Check sheet for the modelled part. Datum: model origin and axes. Units: mm. Face numbers are marked on the shaded views. A direction names the side the tool comes from. Coordinates: 2 decimals unless noted, no trailing zeros. Write each loop counter-clockwise with the first axis right and the second up, starting at its lowest first coordinate (ties: lowest second). Pieces come first, ordered by that corner, then holes. Notation, with made-up numbers: (82.25, -33.5) -> (102.25, -33.5) arc R13 ccw to (102.25, -17.5) -> close; hole circle Ø11 at (-37, -30.5). An arc over 180 degrees is marked (long way). One line per item, written item: value. Start each with the question number.
1) Set-up check for the marked faces 1, 2 and 3: record each of +Z, -Z, +X, -X, +Y, -Y from which the full face is reachable in a straight line by a thin tool's end or side.
2) Draft check along X on the marked faces 4, 5, 6 and 7. Enter one of: +X half, -X half, draft (parallel to the pull), parting line (faces both ways), or undercut.
3) Gauge pin test, flat ends, axial feed: P1, Ø8, axis at y = -39.5, z = 43.5, coming from the -X side; P2, Ø1, axis at y = -33, z = 13, coming from the +X side; P3, Ø12, axis at y = 5, z = 49.5, coming from the +X side; P4, Ø1, axis at x = -4.5, z = 30.5, coming from the -Y side. Record the tip position at first contact, or that the pin passes through.
4) Sectioned sample at A-A on z = 25. Enter the section's corners in (x, y), plus the area to 3 significant figures.
5) Sectioned sample at B-B on x = 32. Enter the section's corners in (y, z), plus the area to 3 significant figures.
6) Sectioned sample at D-D on x = -22. Enter the section's corners in (y, z), plus the area to 3 significant figures.
7) Sectioned sample at C-C on y = -16. Enter the section's corners in (x, z), plus the area to 3 significant figures.
8) Scan lines: line 1 along Y through (x, z) = (-32, 10); line 2 along X through (y, z) = (-11, 25); line 3 along X through (y, z) = (48, 12). Record each from-to range of solid material in increasing order. Write a range as [from, to].
```python
from build123d import *

# Parameters (mm, degrees)
ESQUISSE1_W                  = 80
ESQUISSE1_H                  = 112
BOSS_EXTRU_1_DEPTH           = 100
ESQUISSE4_R                  = 2.5
ENL_V_MAT_EXTRU_2_DEPTH      = 100
ENL_V_MAT_EXTRU_2_DEPTH_BACK = 1
BOSS_EXTRU_2_DEPTH           = 112
BOSS_EXTRU_4_DEPTH           = 112
ENL_V_MAT_EXTRU_6_DEPTH      = 112
ESQUISSE16_R                 = 4.25
ENL_V_MAT_EXTRU_7_DEPTH      = 112
ESQUISSE15_R                 = 4.25
ENL_V_MAT_EXTRU_10_DEPTH     = 112
CONG_1_R                     = 10
CONG_2_R                     = 5
ESQUISSE17_R                 = 4.5
ENL_V_MAT_EXTRU_12_DEPTH     = 112


with BuildPart() as part:
    # Esquisse1 → Boss.-Extru.1 (new body)
    with BuildSketch(Plane.XY):
        Rectangle(ESQUISSE1_W, ESQUISSE1_H)
    extrude(amount=BOSS_EXTRU_1_DEPTH)

    # Esquisse4 → Enlèv. mat.-Extru.2 (cut, two sides)
    with BuildSketch(Plane.XY) as enl_v_mat_extru_2_sk:
        with Locations((-32, 47.99765818)):
            Circle(ESQUISSE4_R)
        with Locations((32, 48)):
            Circle(ESQUISSE4_R)
        with Locations((-32, -48)):
            Circle(ESQUISSE4_R)
        with Locations((32, -48)):
            Circle(ESQUISSE4_R)
    extrude(amount=ENL_V_MAT_EXTRU_2_DEPTH, mode=Mode.SUBTRACT)
    extrude(enl_v_mat_extru_2_sk.sketch, amount=-ENL_V_MAT_EXTRU_2_DEPTH_BACK, mode=Mode.SUBTRACT)

    # Esquisse11 → Boss.-Extru.2 (add)
    with BuildSketch(Plane(origin=(0, 56, 0), x_dir=(1, 0, 0), z_dir=(0, 1, 0))):
        Polygon((-60, -65), (0, -5), (60, -65), align=None)
    extrude(amount=-BOSS_EXTRU_2_DEPTH)

    # Esquisse13 → Boss.-Extru.4 (add)
    with BuildSketch(Plane(origin=(0, 56, 0), x_dir=(1, 0, 0), z_dir=(0, 1, 0))):
        Polygon((-60, -65), (-40, -85), (-40, -65), align=None)
        Polygon((60, -65), (40, -85), (40, -65), align=None)
    extrude(amount=-BOSS_EXTRU_4_DEPTH)

    # Esquisse14 → Enlèv. mat.-Extru.6 (cut)
    with BuildSketch(Plane(origin=(0, 56, 0), x_dir=(1, 0, 0), z_dir=(0, 1, 0))):
        Polygon((-50, -75), (0, -25), (50, -75), (40, -85), (40, -100), (-40, -100), (-40, -85), align=None)
    extrude(amount=-ENL_V_MAT_EXTRU_6_DEPTH, mode=Mode.SUBTRACT)

    # Esquisse16 → Enlèv. mat.-Extru.7 (cut)
    with BuildSketch(Plane(origin=(2.5, 0, 2.5), x_dir=(-0.707106781, 0, 0.707106781), z_dir=(-0.707106781, 0, -0.707106781))):
        with Locations((74.388347648, 36)):
            Circle(ESQUISSE16_R)
        with Locations((74.388347648, -36)):
            Circle(ESQUISSE16_R)
    extrude(amount=-ENL_V_MAT_EXTRU_7_DEPTH, mode=Mode.SUBTRACT)

    # Esquisse15 → Enlèv. mat.-Extru.10 (cut)
    with BuildSketch(Plane(origin=(-2.5, 0, 2.5), x_dir=(-0.707106781, 0, -0.707106781), z_dir=(0.707106781, 0, -0.707106781))):
        with Locations((-74.388347648, 36)):
            Circle(ESQUISSE15_R)
        with Locations((-74.388347648, -36)):
            Circle(ESQUISSE15_R)
    extrude(amount=-ENL_V_MAT_EXTRU_10_DEPTH, mode=Mode.SUBTRACT)

    # Congé1
    cong_1_edges = [part.edges().sort_by_distance(p)[0] for p in [
        (-55, -56, 70),
        (-55, 56, 70),
        (55, 56, 70),
        (55, -56, 70),
    ]]
    fillet(cong_1_edges, radius=CONG_1_R)

    # Congé2
    cong_2_edges = [part.edges().sort_by_distance(p)[0] for p in [
        (40, -56, 22.5),
        (-40, -56, 22.5),
        (-40, 56, 22.5),
        (40, 56, 22.5),
    ]]
    fillet(cong_2_edges, radius=CONG_2_R)

    # Esquisse17 → Enlèv. mat.-Extru.12 (cut)
    with BuildSketch(Plane(origin=(0, 56, 0), x_dir=(1, 0, 0), z_dir=(0, 1, 0))):
        with Locations((0, -25)):
            Circle(ESQUISSE17_R)
    extrude(amount=-ENL_V_MAT_EXTRU_12_DEPTH, mode=Mode.SUBTRACT)


solid = part.part
```
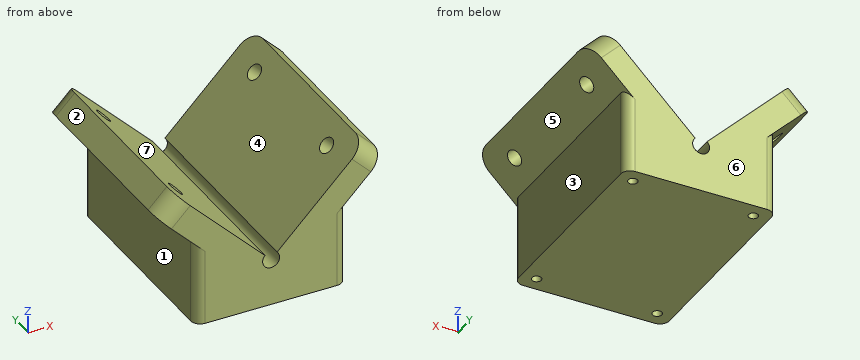
Answers:
1. face 1: -Z, -X, +Y, -Y
1. face 2: +Z, -X, +Y, -Y
1. face 3: -Z, +X, +Y, -Y
2. face 4: undercut
2. face 5: +X half
2. face 6: draft
2. face 7: undercut
3. P1: stops at x = -42.5
3. P2: stops at x = 40
3. P3: stops at x = 50.5
3. P4: passes through
4. outline: (-40, -51) arc R5 ccw to (-35, -56) -> (-4.5, -56) -> (-4.5, 56) -> (-35, 56) arc R5 ccw to (-40, 51) -> close; (4.5, -56) -> (35, -56) arc R5 ccw to (40, -51) -> (40, 51) arc R5 ccw to (35, 56) -> (4.5, 56) -> close; hole circle Ø5 at (-32, -48); hole circle Ø5 at (-32, 48); hole circle Ø5 at (32, -48); hole circle Ø5 at (32, 48)
4. area: 7,850 mm2
5. outline: (-56, 0) -> (-50.5, 0) -> (-50.5, 37) -> (-45.5, 37) -> (-45.5, 0) -> (45.5, 0) -> (45.5, 37) -> (50.5, 37) -> (50.5, 0) -> (56, 0) -> (56, 57) -> (-56, 57) -> close
5. area: 6,010 mm2
6. outline: (-56, 0) -> (56, 0) -> (56, 47) -> (-56, 47) -> close
6. area: 5,260 mm2
7. outline: (-60, 65) -> (-40, 45) -> (-40, 0) -> (40, 0) -> (40, 45) -> (60, 65) -> (50, 75) -> (3.18, 28.18) arc R4.5 cw (long way) to (-3.18, 28.18) -> (-50, 75) -> close
7. area: 4,150 mm2
8. line 1: y = [-56, -50.5], [-45.5, 45.5], [50.5, 56]
8. line 2: x = [-40, -4.5], [4.5, 40]
8. line 3: x = [-40, -34.5], [-29.5, 29.5], [34.5, 40]
